Can you work these out from the drawing? Everything is in mm from the part's minimum corner. Coordinates: 2 decimals unless noted, no trailing zeros. Order: outer loops, then holes, each group sorted by start corner. A loop starts at its lowest first (then second) coordinate and runs counter-clockwise, first axis right, second up. Notation, with made-up numbers: (24, 62) -> (71, 62) arc R16 cw to (71, 89) -> close; hole circle Ø10 at (31, 49). An arc over 180 degrees is marked (long way). Put each result on its own line as item: value. Start each with the question number.
Q1. Will these pins go through, and if not, where does the flat tip stop? pin 1 (1.5 mm diameter, centred on y = 9.5, z = 22, fed in from -X); pin 2 (2 mm diameter, centred on y = 9, z = 64.5, fed in from +X); pin 3 (9.5 mm diameter, centred on x = 13, y = 11, fed in from -Z); pin 4 (8 mm diameter, centred on y = 4, z = 45.5, fed in from +X).
Q2. Please list where these lines run through material, in increasing order: line 1 along Y through (x, z) = (11, 5.5); line 2 along X through (y, z) = (10, 14.25); line 3 along X through (y, z) = (10, 11.75).
Q3. If we section it at C-C (z = 108): Please give me the cut outline in (x, y).
Q4. If we section it at B-B (x = 9): Please give me the cut outline in (y, z).
Q5. If we section it at D-D (y = 3.75): Please give me the cut outline in (x, z), and give its area (3 significant figures).
Q6. If we section it at A-A (y = 10): Please give me the cut outline in (x, z), and give its area (3 significant figures).
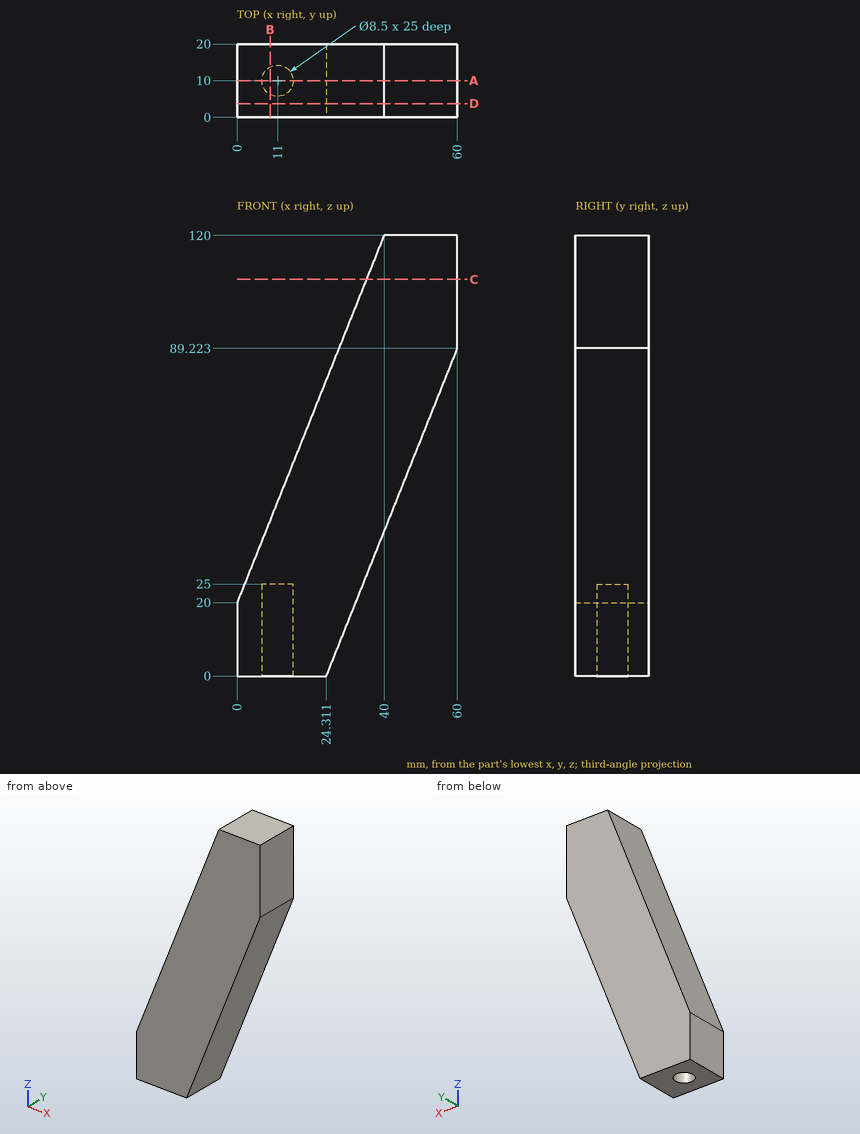
The answers:
1. pin 1: x = 0.5
1. pin 2: x = 50.51
1. pin 3: z = 0
1. pin 4: x = 44.11
2. line 1: 0 to 5.75, 14.25 to 20
2. line 2: 0 to 6.75, 15.25 to 30.01
2. line 3: 0 to 6.75, 15.25 to 29.01
3. outline: (35.2, 0) -> (60, 0) -> (60, 20) -> (35.2, 20) -> close
4. outline: (0, 0) -> (6.25, 0) -> (6.25, 25) -> (13.75, 25) -> (13.75, 0) -> (20, 0) -> (20, 42.5) -> (0, 42.5) -> close
5. outline: (0, 0) -> (24.31, 0) -> (60, 89.22) -> (60, 120) -> (40, 120) -> (0, 20) -> close
5. area: 3,610 mm^2
6. outline: (0, 0) -> (6.75, 0) -> (6.75, 25) -> (15.25, 25) -> (15.25, 0) -> (24.31, 0) -> (60, 89.22) -> (60, 120) -> (40, 120) -> (0, 20) -> close
6. area: 3,400 mm^2
